from build123d import *

# Parameters (mm, degrees)
SKETCH1_R           = 25
BOSS_EXTRUDE1_DEPTH = 40
SKETCH2_R           = 20
CUT_EXTRUDE1_DEPTH  = 70
SKETCH9_R           = 2.5
BOSS_EXTRUDE2_DEPTH = 20
SKETCH3_R           = 40
BOSS_EXTRUDE3_DEPTH = 20
SKETCH4_R           = 25
BOSS_EXTRUDE4_DEPTH = 20
SKETCH5_R           = 20
BOSS_EXTRUDE5_DEPTH = 20
SKETCH6_R           = 15
BOSS_EXTRUDE6_DEPTH = 20
SKETCH7_R           = 10
BOSS_EXTRUDE7_DEPTH = 20
SKETCH8_R           = 5
BOSS_EXTRUDE8_DEPTH = 20


with BuildPart() as part:
    # Sketch1 → Boss-Extrude1 (new body)
    with BuildSketch(Plane(origin=(0, 0, 0), x_dir=(0, 0, -1), z_dir=(1, 0, 0))):
        Circle(SKETCH1_R)
    extrude(amount=BOSS_EXTRUDE1_DEPTH)

    # Sketch2 → Cut-Extrude1 (cut)
    with BuildSketch(Plane(origin=(0, 0, 0), x_dir=(0, 0, -1), z_dir=(1, 0, 0))):
        Circle(SKETCH2_R)
    extrude(amount=CUT_EXTRUDE1_DEPTH, mode=Mode.SUBTRACT)

    # Sketch3 → Boss-Extrude3 (add)
    with BuildSketch(Plane(origin=(40, 0, 0), x_dir=(0, 0, -1), z_dir=(1, 0, 0))):
        Circle(SKETCH3_R)
    extrude(amount=BOSS_EXTRUDE3_DEPTH)

    # Sketch4 → Boss-Extrude4 (add)
    with BuildSketch(Plane(origin=(60, 0, 0), x_dir=(0, 0, -1), z_dir=(1, 0, 0))):
        Circle(SKETCH4_R)
    extrude(amount=BOSS_EXTRUDE4_DEPTH)

    # Sketch5 → Boss-Extrude5 (add)
    with BuildSketch(Plane(origin=(80, 0, 0), x_dir=(0, 0, -1), z_dir=(1, 0, 0))):
        Circle(SKETCH5_R)
    extrude(amount=BOSS_EXTRUDE5_DEPTH)

    # Sketch6 → Boss-Extrude6 (add)
    with BuildSketch(Plane(origin=(100, 0, 0), x_dir=(0, 0, -1), z_dir=(1, 0, 0))):
        Circle(SKETCH6_R)
    extrude(amount=BOSS_EXTRUDE6_DEPTH)

    # Sketch7 → Boss-Extrude7 (add)
    with BuildSketch(Plane(origin=(120, 0, 0), x_dir=(0, 0, -1), z_dir=(1, 0, 0))):
        Circle(SKETCH7_R)
    extrude(amount=BOSS_EXTRUDE7_DEPTH)



with BuildPart() as body_2:
    # Sketch9 → Boss-Extrude2 (new body)
    with BuildSketch(Plane(origin=(160, 0, 0), x_dir=(0, 0, -1), z_dir=(1, 0, 0))):
        Circle(SKETCH9_R)
    extrude(amount=BOSS_EXTRUDE2_DEPTH)


with BuildPart() as part_1:
    add(part.part)

    add(body_2.part)  # Boss-Extrude8 merges body 2
    # Sketch8 → Boss-Extrude8 (add)
    with BuildSketch(Plane(origin=(140, 0, 0), x_dir=(0, 0, -1), z_dir=(1, 0, 0))):
        Circle(SKETCH8_R)
    extrude(amount=BOSS_EXTRUDE8_DEPTH)


solid = part_1.part
Build history of the part. All positions in model axes, mm. A direction names the side the tool comes from. Coordinates: 2 decimals unless noted, no trailing zeros. Write each loop counter-clockwise with the first axis right and the second up, starting at its lowest first coordinate (ties: lowest second). Pieces come first, ordered by that corner, then holes.
(1) Cut at C-C on x = 64.5. List the corners of the cut face in (y, z).
(2) Cut at A-A on z = -32. List the corners of the cut face in (x, y).
(3) Pin check, flat tips, straight feed: pin 1 Ø12 at (y, z) = (4.5, 7.5) entering from -X; pin 2 Ø1 at (x, y) = (61, -1) entering from +Z (3 decimals); pin 3 Ø8 at (y, z) = (14, -25) entering from +X. Stop position of each tip, or through.
(4) 3-axis set-ups, long thin cutter, end or side, ignore diameter. For faces 1 (the cylindrical face through (49.86, -39.05, 8.67)), 2 (the cylindrical face through (109.86, 0.66, 14.985)), 3 (the flat face through (40, 18.34, -17.22)): which of +Z, -Z, +X, -X, +Y, -Y reach the whole face in a straight line?
(5) Drill centre lines: line 1 (Y direction, x = 30, z = 0); line 2 (X direction, y = 9, z = 25); line 3 (X direction, y = 5, z = 6). Where is each one in solid material? Low to high.
(6) Cut at D-D on x = 30. List the corners of the cut face in (y, z), and give its area (3 significant figures).
(7) Mould opens along Z. For faces 4 (the cylindrical face through (19.72, -19.524, 4.336)), 5 (the cylindrical face through (19.72, 7.509, -23.846)), 6 (the flat face through (40, 0, 0)), 7 (the flat face through (0, 17, 11)) say: pulls with the +Z half, pulls with the -Z half, needs draft (parallel to the pull), parting line crosses it, or undercut.
Working result:
1. outline: circle Ø50 at (0, 0)
2. outline: (40, -24) - (60, -24) - (60, 24) - (40, 24) - close
3. pin 1: stops at x = 40
3. pin 2: stops at z = 24.995
3. pin 3: stops at x = 80
4. face 1: +X, -X
4. face 2: +X
4. face 3: -X
5. line 1: y = -25 to -20, 20 to 25
5. line 2: x = 40 to 60
5. line 3: x = 40 to 140
6. outline: circle Ø50 at (0, 0); hole circle Ø40 at (0, 0)
6. area: 707 mm2
7. face 4: undercut
7. face 5: parting line crosses it
7. face 6: undercut
7. face 7: needs draft
